Check sheet for the modelled part. Datum: model origin and axes. Units: mm. Face numbers are marked on the shaded views. A direction names the side the tool comes from. Round coordinates to 2 decimals unless told otherwise and drop trailing zeros. Write each loop counter-clockwise with the first axis right and the second up, starting at its lowest first coordinate (ties: lowest second). Pieces come first, ordered by that corner, then holes.
Item 1: Go/stop test with a flat-tipped pin: pin 1 Ø0.8 at (x, z) = (19, 4) entering from -Y. Record where the tip stops, or that it passes through.
Item 2: Cross-section at A-A on y = -5.5. Enter the section's corners in (x, z), plus the area to 3 significant figures.
Item 3: Tool access check on the marked faces 4, 5 and 6. Record the directions out of +Z, -Z, +X, -X, +Y, -Y that give a thin tool (end or side, any length) a straight path to the whole face; none if there is none.
Item 4: Release check for a two-part mould opening along X. For the marked faces 1, 2 and 3 record: +X half, -X half, draft (parallel to the pull), parting line (faces both ways), or undercut.
Item 5: Cross-section at B-B on y = 7.25. Enter the section's corners in (x, z).
Item 6: Material ranges on line 1 (X direction, y = -3.25, z = 4); line 2 (X direction, y = -2.25, z = 1.75); line 3 (Y direction, x = -19, z = 3.25), recorded low to high.
Item 7: Cross-section at C-C on x = 12.5. Enter the section's corners in (y, z).
Autodesk Inventor part; units mm, degrees
ref_plane "YZ Plane" through (0, 0, 0) normal (1, 0, 0) x (0, 1, 0)
ref_plane "XZ Plane" through (0, 0, 0) normal (0, 1, 0) x (-1, 0, 0)
ref_plane "XY Plane" through (0, 0, 0) normal (0, 0, 1) x (1, 0, 0)
sketch "Sketch1" plane through (0, 0, 0) normal (0, 0, 1) x (1, 0, 0)
  line L0 (0, 0) -> (-17.7, 0)
  line L1 (-20, -9.2) -> (-18.6, -9.2)
  line L2 (-18.6, -9.2) -> (-18.6, -13.2)
  line L3 (-18.6, -13.2) -> (-25, -13.2)
  line L4 (-25, -13.2) -> (-25, 3.7158)
  arc A0 (-18.6667, 8.5348) -> (-25, 3.7158) centre (-20, 3.7158) ccw
  arc A1 (-18.6667, 8.5348) -> (0, 6) centre (0, 76) ccw
  line L5 (0, 0) -> (0, 6) construction
  line L6 (-18.5, -0.8) -> (-18.5, -3)
  line L7 (-18.5, -3) -> (-20, -3)
  line L8 (-20, -3) -> (-20, -9.2)
  arc A2 (-17.7, 0) -> (-18.5, -0.8) centre (-18.5, 0) ccw
  line L9 (0, 0) -> (17.7, 0)
  line L10 (20, -9.2) -> (18.6, -9.2)
  line L11 (18.6, -9.2) -> (18.6, -13.2)
  line L12 (18.6, -13.2) -> (25, -13.2)
  line L13 (25, -13.2) -> (25, 3.7158)
  arc A3 (25, 3.7158) -> (18.6667, 8.5348) centre (20, 3.7158) ccw
  arc A4 (0, 6) -> (18.6667, 8.5348) centre (0, 76) ccw
  line L14 (18.5, -0.8) -> (18.5, -3)
  line L15 (18.5, -3) -> (20, -3)
  line L16 (20, -3) -> (20, -9.2)
  arc A5 (18.5, -0.8) -> (17.7, 0) centre (18.5, 0) ccw
  line L17 (-20, 8.7158) -> (20, 8.7158) construction
  dimension "d0" = 6
  dimension "d4" = 6.2
  dimension "d5" = 1.5
  dimension "d7" = 4
  dimension "d9" = 5
  dimension "d10" = 70
  dimension "d11" = 5
  dimension "d12" = 0.8
  dimension "d13" = 3
  dimension "d18" = 1.4
  dimension "d20" = 18.5
  dimension "d26" = 8.7158
extrude "Extrusion1" add sketch "Sketch1" along normal blind 6
fillet "Fillet1" radius 2 4 edges at (-18.6, -13.2, 3) (-25, -13.2, 3) (18.6, -13.2, 3) (25, -13.2, 3)
fillet "Fillet2" radius 0.5 2 edges at (-18.6, -9.2, 3) (18.6, -9.2, 3)
fillet "Fillet3" radius 0.5 4 edges at (-18.5, -0.8, 3) (-17.7, 0, 3) (17.7, 0, 3) (18.5, -0.8, 3)
sketch "Sketch2" plane through (0, 0, 6) normal (0, 0, 1) x (1, 0, 0)
  arc A0 (1, 0.25) -> (-1, 0.25) centre (0, 0.25) ccw
  line L0 (-17.3, 0) -> (17.3, 0)
  line L1 (-1, 0.25) -> (-1, 0)
  line L2 (1, 0.25) -> (1, 0)
  point P0 (0, 0)
  point P1 (0, 0)
  dimension "d21" = 0.25
  dimension "d25" = 1
extrude "Extrusion2" cut sketch "Sketch2" against normal through all
fillet "Fillet4" radius 0.5 2 edges at (-1, 0, 3) (1, 0, 3)
equation "\"d5\" = GripLength"
equation "\"d20\" = 0.5 * BattECOD - GripLength"
properties part number "Twist Lock"
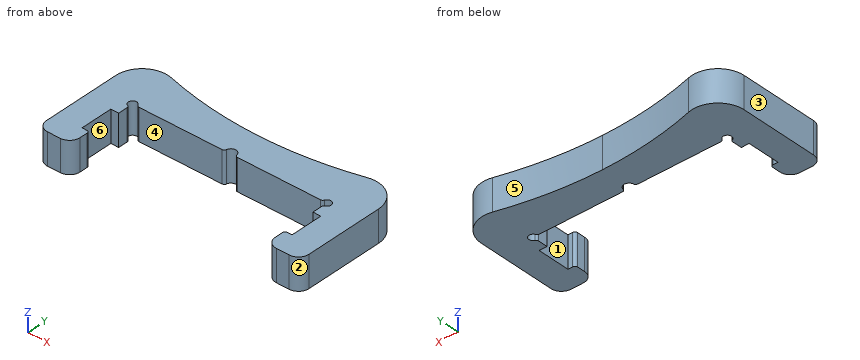
Response values:
1. pin 1: stops at y = -12.8
2. outline: (-25, 0) - (-20, 0) - (-20, 6) - (-25, 6) - close; (20, 0) - (25, 0) - (25, 6) - (20, 6) - close
2. area: 60.0 mm2
3. face 4: +Z, -Z, -Y
3. face 5: +Z, -Z, +Y
3. face 6: +Z, -Z
4. face 1: undercut
4. face 2: +X half
4. face 3: -X half
5. outline: (-23.54, 0) - (-13.17, 0) - (-13.17, 6) - (-23.54, 6) - close; (13.17, 0) - (23.54, 0) - (23.54, 6) - (13.17, 6) - close
6. line 1: x = -25 to -20, 20 to 25
6. line 2: x = -25 to -18.5, 18.5 to 25
6. line 3: y = -12.4 to -9.21, -3 to -0.62, 0.62 to 8.61
7. outline: (0, 0) - (7.13, 0) - (7.13, 6) - (0, 6) - close
